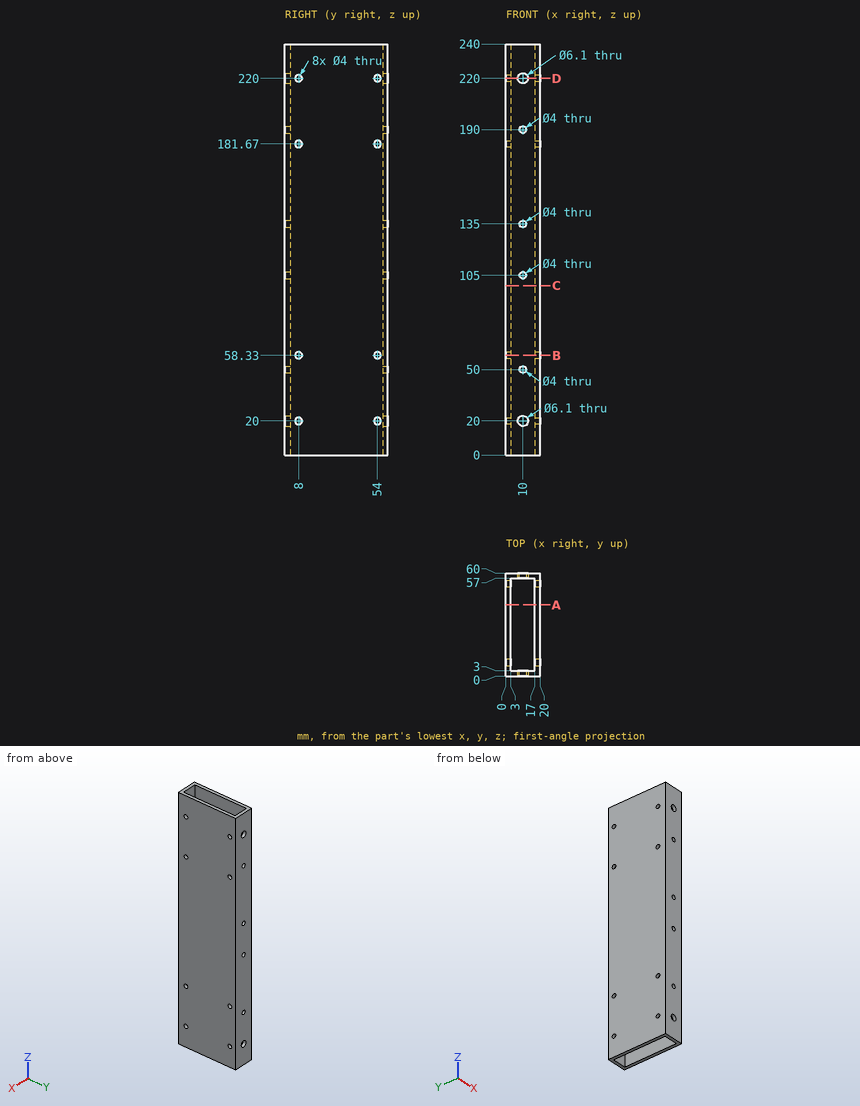
Input: dimensioned drawing with shaded views. Units: mm. Origin: part minimum x, y, z. Coordinates: 2 decimals unless noted, no trailing zeros. Loops run counter-clockwise (first coordinate to the right, second up) from the corner with the lowest first, then second, coordinate; pieces in that order, holes last. Notation, with made-up numbers: M 38,40.25 L 92,40.25 A8 cw 92,54.25 Z; hole C -19,53.5 d5. An arc over 180 degrees is marked long. Use a Markdown table: item, result. Add a question column.
1) Line query: L1, parallel to Y at x = 17.65, z = 181.67; L2, parallel to X at y = 40.5, z = 171; L3, parallel to Y at x = 5.25, z = 168.5. Output: solid intervals per line, ascending. Write a range as from..to.
2) Section D-D, the plane z = 220. Give the number of separate pieces and of enclosed holes in the cut face, plus the area to 3 significant figures.
3) Pin query (flat end, axial travel): P1, Ø5.5, axis at x = 10, z = 220, coming from the -Y side. Return the tip coordinate at first contact, or that it passes through.
4) Section A-A, the plane y = 41.5. Return the cut outline in (x, z).
5) Section C-C, the plane z = 99. Return the cut outline in (x, y), plus the area to 3 significant figures.
6) Section B-B, the plane z = 58.33. Return the cut outline in (x, y).
Answer below:
| question | item | result |
|---|---|---|
| 1 | L1 | 0..6, 10..52, 56..60 |
| 1 | L2 | 0..3, 17..20 |
| 1 | L3 | 0..3, 57..60 |
| 2 | separate pieces | 6 |
| 2 | enclosed holes | 0 |
| 2 | area | 359 mm2 |
| 3 | P1 | through |
| 4 | outline | M 0,0 L 3,0 L 3,240 L 0,240 Z; M 17,0 L 20,0 L 20,240 L 17,240 Z |
| 5 | outline | M 0,0 L 20,0 L 20,60 L 0,60 Z; hole M 3,3 L 17,3 L 17,57 L 3,57 Z |
| 5 | area | 444 mm2 |
| 6 | outline | M 0,0 L 20,0 L 20,6 L 17,6 L 17,3 L 3,3 L 3,6 L 0,6 Z; M 0,10 L 3,10 L 3,52 L 0,52 Z; M 0,56 L 3,56 L 3,57 L 17,57 L 17,56 L 20,56 L 20,60 L 0,60 Z; M 17,10 L 20,10 L 20,52 L 17,52 Z |
